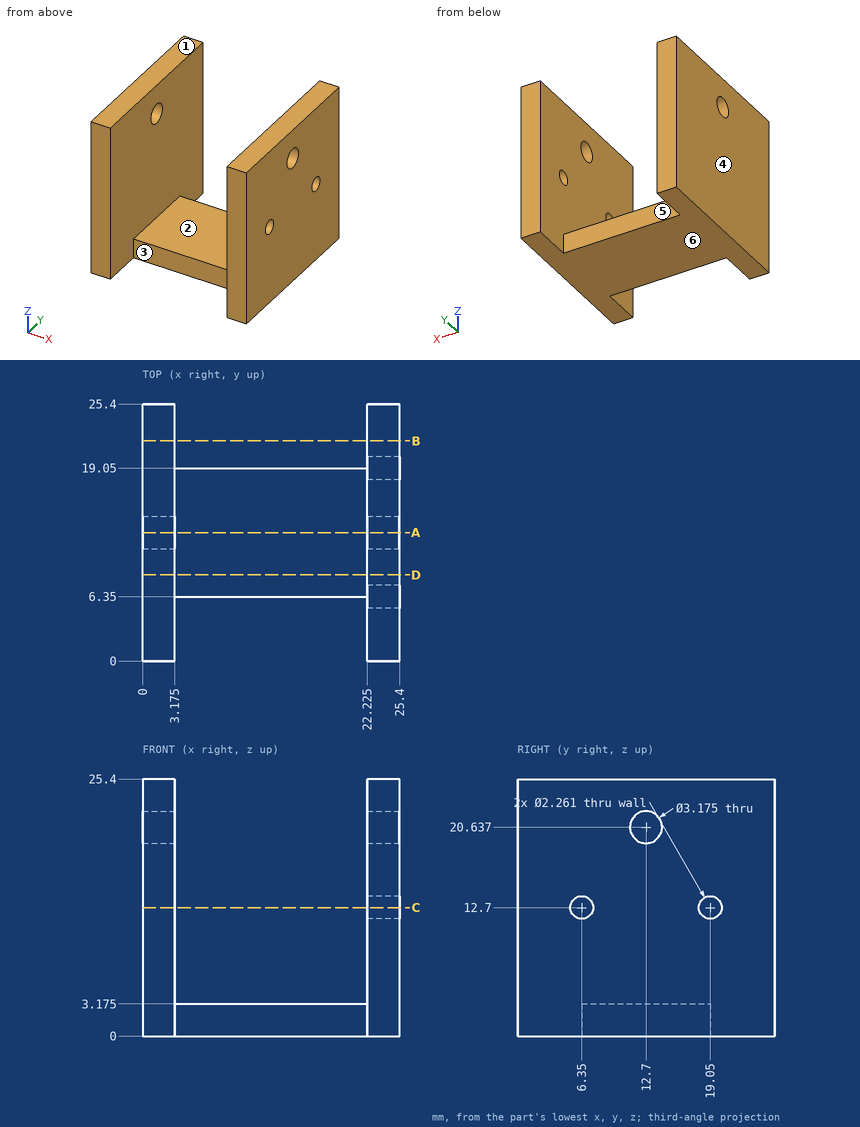
Print and shaded views of the part. All mm, measured from the part's lowest x, y and z. A direction names the side the tool comes from. Coordinates: 2 decimals unless noted, no trailing zeros. Loops run counter-clockwise (first coordinate to the right, second up) from the corner with the lowest first, then second, coordinate; pieces in that order, holes last. Notation, with made-up numbers: M 2.25,15.5 L 58.25,15.5 A15 cw 58.25,21.5 Z; hole C 56,-13.5 d6. An arc over 180 degrees is marked long. Use a Markdown table: item, result. Add a question column.
Q1. Mould opens along X. For the marked faces 4, 5 and 6 say: +X half, -X half, draft (parallel to the pull), parting line (faces both ways), or undercut.
Q2. Cut at C-C (z = 12.7). Write the cut outline in (x, y) (1 decimal).
Q3. Which spindle directions (+Z, -Z, +X, -X, +Y, -Y) get a long thin tool onto all of the face, cutting with end or side? Do the marked faces 1, 2 and 3. Say none if no direction does.
Q4. Cut at B-B (y = 21.75). Write the cut outline in (x, z) (1 decimal).
Q5. Pin check, flat tips, straight feed: P1, Ø1.8, axis at y = 6.35, z = 12.7, coming from the -X side; P2, Ø2, axis at y = 19.05, z = 12.7, coming from the +X side (1 decimal); P3, Ø1.6, axis at x = 10, z = 1, coming from the +Y side; P4, Ø1, axis at x = 5.5, y = 12, coming from the +Z side (1 decimal). Stop position of each tip, or through.
Q6. Probe L1, parallel to X at y = 12.25, z = 4 (1 decimal); L2, parallel to Y at x = 13.5, z = 1; L3, parallel to Z at x = 16.25, y = 14.5 (1 decimal). List the from-to ranges inside material, lowest first.
Q7. Cut at D-D (y = 8.5). Write the cut outline in (x, z) (1 decimal).
Q8. Cut at A-A (y = 12.7). Give the number of separate pieces and of enclosed holes in the cut face.
Worked out:
| question | item | result |
|---|---|---|
| 1 | face 4 | -X half |
| 1 | face 5 | undercut |
| 1 | face 6 | draft |
| 2 | outline | M 0,0 L 3.2,0 L 3.2,25.4 L 0,25.4 Z; M 22.2,0 L 25.4,0 L 25.4,5.2 L 22.2,5.2 Z; M 22.2,7.5 L 25.4,7.5 L 25.4,17.9 L 22.2,17.9 Z; M 22.2,20.2 L 25.4,20.2 L 25.4,25.4 L 22.2,25.4 Z |
| 3 | face 1 | +Z, +X, -X, +Y, -Y |
| 3 | face 2 | +Z, +Y, -Y |
| 3 | face 3 | +Z, -Z, -Y |
| 4 | outline | M 0,0 L 3.2,0 L 3.2,25.4 L 0,25.4 Z; M 22.2,0 L 25.4,0 L 25.4,25.4 L 22.2,25.4 Z |
| 5 | P1 | stops at x = 0 |
| 5 | P2 | stops at x = 3.2 |
| 5 | P3 | stops at y = 19.05 |
| 5 | P4 | stops at z = 3.2 |
| 6 | L1 | x = 0 to 3.2, 22.2 to 25.4 |
| 6 | L2 | y = 6.35 to 19.05 |
| 6 | L3 | z = 0 to 3.2 |
| 7 | outline | M 0,0 L 25.4,0 L 25.4,25.4 L 22.2,25.4 L 22.2,3.2 L 3.2,3.2 L 3.2,25.4 L 0,25.4 Z |
| 8 | separate pieces | 3 |
| 8 | enclosed holes | 0 |
